Can you work these out from the drawing? Everything is in mm from the part's minimum corner. Round coordinates to 2 decimals unless told otherwise and drop trailing zeros. Write each loop counter-clockwise with the first axis right and the second up, starting at its lowest first coordinate (ties: lowest second). Pieces come first, ordered by that corner, then holes. Notation, with made-up numbers: M 73,75 L 125,75 A22 ccw 125,95 Z; hole C -30,66 d3. An arc over 180 degrees is marked long. Use a Markdown table: item, result. Add a question column.
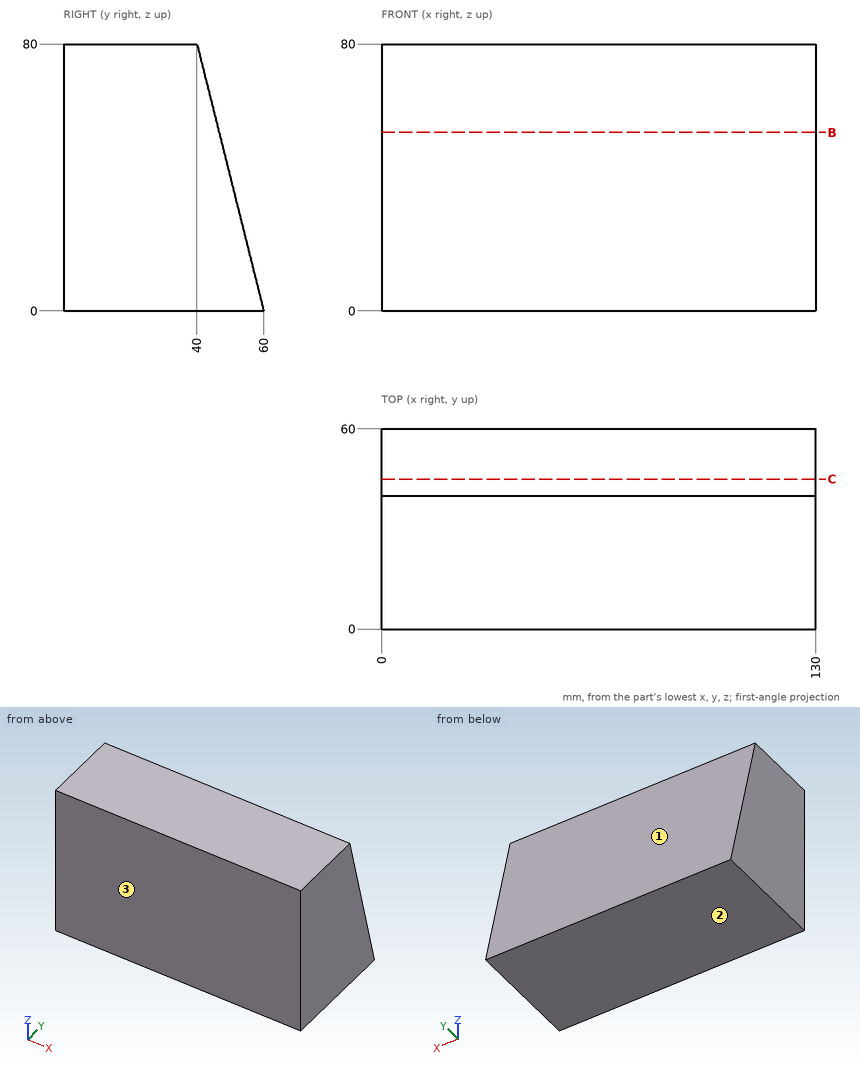
Item 1: I need wall thicknesses on probe 1 along Y at (x, z) = (19, 23); probe 2 along Y at (x, z) = (43, 27). Which ranges of each line are inside material? Lowest first, please. Write a range as from..to.
Item 2: If we mould it in two halves opening along Y, with no side actions, what happens to the marked faces 1, 2 and 3? For each: +Y half, -Y half, draft (parallel to the pull), parting line (faces both ways), or undercut.
Item 3: Imagine slicing it at C-C on y = 45. List the corners of the cut face in (x, z) for me, plus the area to 3 significant figures.
Item 4: For pin 1 Ø5 at (x, z) = (18, 46.5) entering from +Y, with a flat end and sliding along its axis, tell me the tip position at first contact or that it passes through.
Item 5: Imagine slicing it at B-B on z = 53.5. List the corners of the cut face in (x, y) for me (3 decimals), plus the area to 3 significant figures.
The answers:
| question | item | result |
|---|---|---|
| 1 | probe 1 | 0..54.25 |
| 1 | probe 2 | 0..53.25 |
| 2 | face 1 | +Y half |
| 2 | face 2 | draft |
| 2 | face 3 | -Y half |
| 3 | outline | M 0,0 L 130,0 L 130,60 L 0,60 Z |
| 3 | area | 7,800 mm² |
| 4 | pin 1 | y = 49 |
| 5 | outline | M 0,0 L 130,0 L 130,46.625 L 0,46.625 Z |
| 5 | area | 6,060 mm² |
